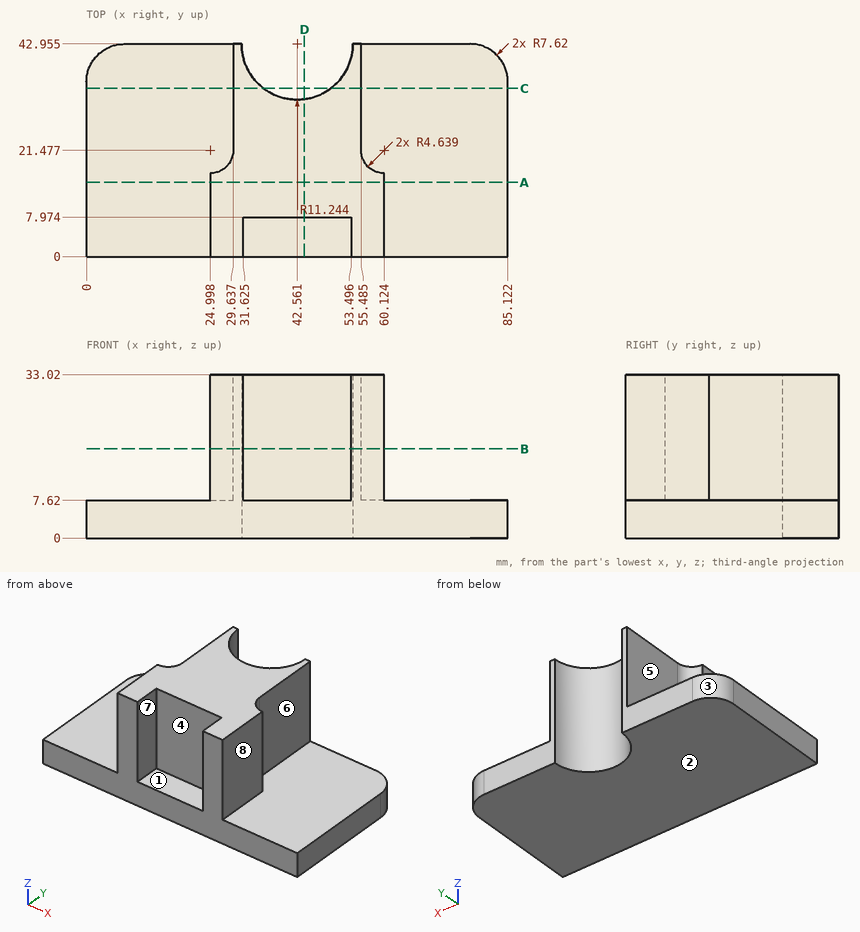
Geometry: see drawing. Coordinates: mm, zero at the bounding-box minimum. A direction names the side the tool comes from. Give positions to 0.01 mm unless a question says otherwise; leave off trailing zeros. Order: outer loops, then holes, each group sorted by start corner. A loop starts at its lowest first (then second) coordinate and runs counter-clockwise, first axis right, second up. Notation, with made-up numbers: (-8, 64) - (12, 64) arc R29 cw to (12, 103) - close; hole circle Ø7 at (5.5, 51). An arc over 180 degrees is marked (long way). Use a Markdown table: item, result.
(1) Section query B-B (z = 18). Output: boundary loops of the cut face in (x, y) (1 decimal).
Computed values:
| item | result |
|---|---|
| outline | (25, 0) - (31.6, 0) - (31.6, 8) - (53.5, 8) - (53.5, 0) - (60.1, 0) - (60.1, 16.8) arc R4.6 cw to (55.5, 21.5) - (55.5, 43) - (53.8, 43) arc R11.2 cw to (31.3, 43) - (29.6, 43) - (29.6, 21.5) arc R4.6 cw to (25, 16.8) - close |
(2) Access query for the marked faces 5, 6, 7 and 8. Directions: +Z, -Z, +X, -X, +Y, -Y. A direction counts if a zero-diameter tool reaches every point of the face in a straight line with its end or side. Return the directions, or none.
Computed values:
| item | result |
|---|---|
| face 5 | +Z, -X, +Y |
| face 6 | +Z, +X, +Y |
| face 7 | +Z, -Y |
| face 8 | +Z, +X, +Y, -Y |
(3) Draft query along X for the marked faces 1, 2, 3 and 4. Return one class per face: released by +X, released by -X, zero draft, split by the parting line, or undercut.
Computed values:
| item | result |
|---|---|
| face 1 | undercut |
| face 2 | zero draft |
| face 3 | released by -X |
| face 4 | undercut |
(4) Pin query (flat end, axial travel): pin 1 (5 mm diameter, centred on y = 37, z = 18, fed in from +X) (1 decimal); pin 2 (5 mm diameter, centred on y = 10.5, z = 22, fed in from -X); pin 3 (4 mm diameter, centred on y = 3.5, z = 20.5, fed in from +X). Return the tip coordinate at first contact, or that it passes through.
Computed values:
| item | result |
|---|---|
| pin 1 | stops at x = 55.5 |
| pin 2 | stops at x = 25 |
| pin 3 | stops at x = 60.12 |
(5) Section query A-A (y = 15). Output: boundary loops of the cut face in (x, z), then the cut area to 3 significant figures.
Computed values:
| item | result |
|---|---|
| outline | (0, 0) - (85.12, 0) - (85.12, 7.62) - (60.12, 7.62) - (60.12, 33.02) - (25, 33.02) - (25, 7.62) - (0, 7.62) - close |
| area | 1,540 mm2 |
(6) Section query C-C (y = 34). Output: boundary loops of the cut face in (x, z) (1 decimal).
Computed values:
| item | result |
|---|---|
| outline | (0, 0) - (35.8, 0) - (35.8, 33) - (29.6, 33) - (29.6, 7.6) - (0, 7.6) - close; (49.4, 0) - (85.1, 0) - (85.1, 7.6) - (55.5, 7.6) - (55.5, 33) - (49.4, 33) - close |
(7) Section query D-D (x = 44). Output: boundary loops of the cut face in (y, z).
Computed values:
| item | result |
|---|---|
| outline | (0, 0) - (31.8, 0) - (31.8, 33.02) - (7.97, 33.02) - (7.97, 7.62) - (0, 7.62) - close |
(8) Line query: line 1 (X direction, y = 3.5, z = 15.5) (1 decimal); line 2 (Z direction, x = 58.5, y = 40); line 3 (X direction, y = 11.5, z = 30.5). Output: solid intervals per line, ascending. Write a range as from..to.
Computed values:
| item | result |
|---|---|
| line 1 | x = 25..31.6, 53.5..60.1 |
| line 2 | z = 0..7.62 |
| line 3 | x = 25..60.12 |
